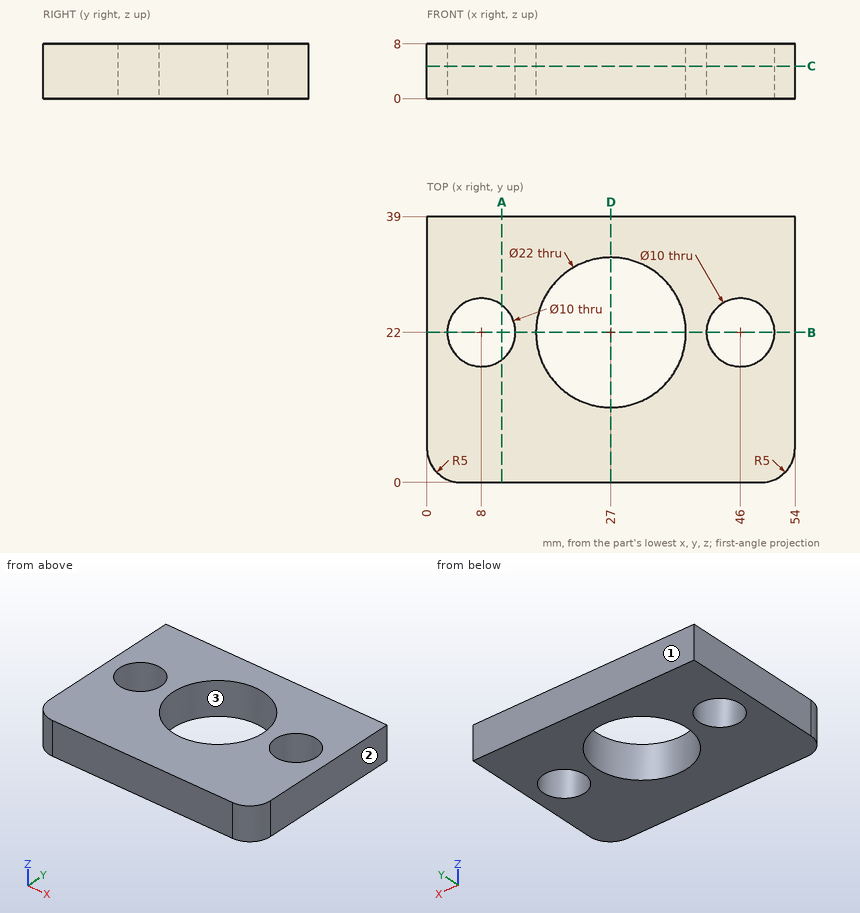
Verification items for this drawing (mm, ordinates from the low corner). Coordinates: 2 decimals unless noted, no trailing zeros. Write each loop counter-clockwise with the first axis right and the second up, starting at its lowest first coordinate (ties: lowest second). Pieces come first, ordered by that corner, then holes. Notation, with made-up numbers: M 13.5,-1.5 L 62.5,-1.5 A26 ccw 62.5,13.5 Z; hole C 58.5,-12 d9. An arc over 180 degrees is marked long. Answer as CSV lines item,"result".
Q1. Cross-section at C-C (z = 4.75). Record the boundary of the cut face in (x, y), then the cut area to 3 significant figures.
Check result:
outline,"M 0,5 A5 ccw 5,0 L 49,0 A5 ccw 54,5 L 54,39 L 0,39 Z; hole C 8,22 d10; hole C 27,22 d22; hole C 46,22 d10"
area,"1,560 mm^2"
Q2. Mould release check, pull along X, two halves, no side actions. Record for the marked faces 1, 2 and 3: released by +X, released by -X, zero draft, split by the parting line, or undercut.
Check result:
face 1,"zero draft"
face 2,"released by +X"
face 3,"undercut"
Q3. Material ranges on probe 1 along Y at (x, z) = (8, 5); probe 2 along Y at (x, z) = (27, 3.75); probe 3 along X at (y, z) = (18, 7), recorded low to high. Write a range as from..to.
Check result:
probe 1,"0..17, 27..39"
probe 2,"0..11, 33..39"
probe 3,"0..5, 11..16.75, 37.25..43, 49..54"
Q4. Cross-section at D-D (x = 27). Record the boundary of the cut face in (y, z), then the cut area to 3 significant figures.
Check result:
outline,"M 0,0 L 11,0 L 11,8 L 0,8 Z; M 33,0 L 39,0 L 39,8 L 33,8 Z"
area,"136 mm^2"
Q5. Cross-section at A-A (x = 11). Record the boundary of the cut face in (y, z).
Check result:
outline,"M 0,0 L 18,0 L 18,8 L 0,8 Z; M 26,0 L 39,0 L 39,8 L 26,8 Z"
Q6. Cross-section at B-B (y = 22). Record the boundary of the cut face in (x, z).
Check result:
outline,"M 0,0 L 3,0 L 3,8 L 0,8 Z; M 13,0 L 16,0 L 16,8 L 13,8 Z; M 38,0 L 41,0 L 41,8 L 38,8 Z; M 51,0 L 54,0 L 54,8 L 51,8 Z"
